The figure shows three views and two pictorial views of one solid part (mm, origin at its lowest corner). Answer the questions. Give positions to 0.01 mm unless a question says otherwise; leave off trailing zeros. Order: outer loops, then holes, each group sorted by start corner. A loop starts at its lowest first (then second) coordinate and runs counter-clockwise, first axis right, second up. Notation, with made-up numbers: (-40, 58) -> (-11, 58) arc R30 cw to (-11, 91) -> close; hole circle Ø2 at (64.5, 35.5). An arc over 180 degrees is marked (long way). One line per item, written item: value. Start each with the question number.
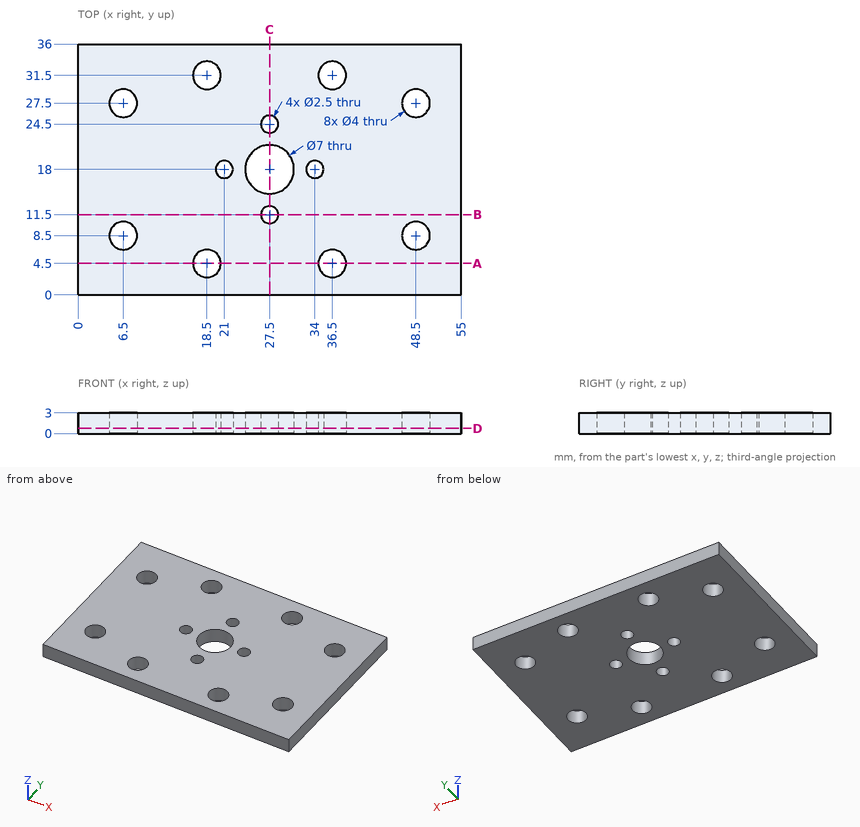
Item 1: Find section A-A on y = 4.5. Write down the section's boundary in (x, z).
Item 2: Flat-ended cylindrical pins translate along their axes: pin 1 (4.5 mm diameter, centred on x = 6.5, y = 8.5, fed in from -Z); pin 2 (3.5 mm diameter, centred on x = 36.5, y = 4.5, fed in from -Z). Find the tip coordinate at first contact, or state that the pin passes through.
Item 3: Find section C-C on x = 27.5. Write down the section's boundary in (y, z), then the cut area to 3 significant figures.
Item 4: Find section D-D on z = 0.75. Count the separate pieces of the cut face and the enclosed holes in it, then the cut area to 3 significant figures.
Item 5: Find section B-B on y = 11.5. Write down the section's boundary in (x, z), then the cut area to 4 significant figures.
Item 6: Find the intervals of material crossed by line 1 (Y direction, x = 18.5, z = 2.3); line 2 (X direction, y = 10, z = 0.95); line 3 (Y direction, x = 27.5, z = 1.8), in increasing order. Write a range as from..to.
Checks:
1. outline: (0, 0) -> (16.5, 0) -> (16.5, 3) -> (0, 3) -> close; (20.5, 0) -> (34.5, 0) -> (34.5, 3) -> (20.5, 3) -> close; (38.5, 0) -> (55, 0) -> (55, 3) -> (38.5, 3) -> close
2. pin 1: z = 0
2. pin 2: through
3. outline: (0, 0) -> (10.25, 0) -> (10.25, 3) -> (0, 3) -> close; (12.75, 0) -> (14.5, 0) -> (14.5, 3) -> (12.75, 3) -> close; (21.5, 0) -> (23.25, 0) -> (23.25, 3) -> (21.5, 3) -> close; (25.75, 0) -> (36, 0) -> (36, 3) -> (25.75, 3) -> close
3. area: 72.0 mm2
4. separate pieces: 1
4. enclosed holes: 13
4. area: 1,820 mm2
5. outline: (0, 0) -> (26.25, 0) -> (26.25, 3) -> (0, 3) -> close; (28.75, 0) -> (55, 0) -> (55, 3) -> (28.75, 3) -> close
5. area: 157.5 mm2
6. line 1: 0..2.5, 6.5..29.5, 33.5..36
6. line 2: 0..5.18, 7.82..47.18, 49.82..55
6. line 3: 0..10.25, 12.75..14.5, 21.5..23.25, 25.75..36
